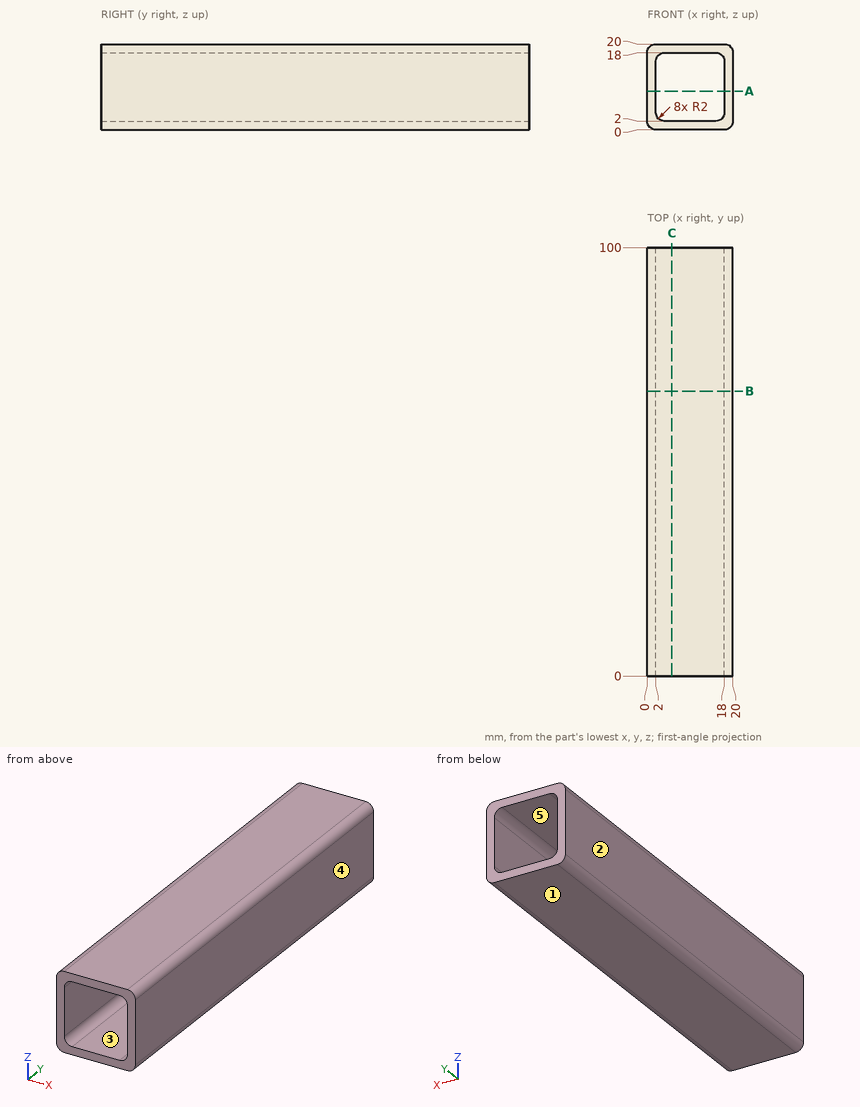
Can you work these out from the drawing? Everything is in mm from the part's minimum corner. A direction names the side the tool comes from. Give positions to 0.01 mm unless a question says otherwise; leave off trailing zeros. Loops run counter-clockwise (first coordinate to the right, second up) from the corner with the lowest first, then second, coordinate; pieces in that order, holes last. Notation, with made-up numbers: M -30.5,-39 L 6.5,-39 A15 ccw 6.5,-29 Z; hole C 62,-2.5 d10. An arc over 180 degrees is marked long. Use CSV: the item, a comma, the result in double quotes. Start each with the question number.
1. Imagine slicing it at B-B, the plane y = 66.5. Write out the boundary of the cut face in (x, z).
2. If we mould it in two halves opening along X, with no side actions, what happens to the marked faces 1, 2 and 3? For each: released by +X, released by -X, zero draft, split by the parting line, or undercut.
3. If I drill on L1, parallel to X at y = 94.5, z = 6; L2, parallel to Z at x = 1.25, y = 63, over which ranges is the centre line in solid material (lowest first)?
4. Imagine slicing it at C-C, the plane x = 5.75. Write out the boundary of the cut face in (y, z), plus the area to 3 significant figures.
5. Imagine slicing it at A-A, the plane z = 9. Write out the boundary of the cut face in (x, y).
6. On a 3-axis mill with a long thin cutter (end or side, diameter ignored), from which of +Z, -Z, +X, -X, +Y, -Y can I reach the whole of each face in a straight line? I mean the marked faces 4 and 5. Say none if no direction works.
Response values:
1,outline,"M 0,2 A2 ccw 2,0 L 18,0 A2 ccw 20,2 L 20,18 A2 ccw 18,20 L 2,20 A2 ccw 0,18 Z; hole M 2,4 A2 ccw 4,2 L 16,2 A2 ccw 18,4 L 18,16 A2 ccw 16,18 L 4,18 A2 ccw 2,16 Z"
2,face 1,"zero draft"
2,face 2,"released by -X"
2,face 3,"undercut"
3,L1,"0 to 2, 18 to 20"
3,L2,"0.15 to 19.85"
4,outline,"M 0,0 L 100,0 L 100,2 L 0,2 Z; M 0,18 L 100,18 L 100,20 L 0,20 Z"
4,area,"400 mm^2"
5,outline,"M 0,0 L 2,0 L 2,100 L 0,100 Z; M 18,0 L 20,0 L 20,100 L 18,100 Z"
6,face 4,"+Z, -Z, +X, +Y, -Y"
6,face 5,"+Y, -Y"
